The model under review builds one solid part; all positions refer to its coordinate system, in mm. A direction names the side the tool comes from. Coordinates: 2 decimals unless noted, no trailing zeros. Write each loop counter-clockwise with the first axis right and the second up, starting at its lowest first coordinate (ties: lowest second). Pieces come first, ordered by that corner, then holes. Notation, with made-up numbers: (89.5, 57) -> (110.5, 57) arc R24 cw to (110.5, 95) -> close; hole circle Ø7 at (-30, 75). An arc over 180 degrees is marked (long way). Write each question's results on one line, items separated by ' | '.
```python
from build123d import *

# Parameters (mm, degrees)
F1_DEPTH      = 508
F7_DEPTH      = 34.6420161514
F7_DEPTH_BACK = 34.6420161514
F8_DEPTH      = 43.3022701892
F8_DEPTH_BACK = 43.3022701892
F9_DEPTH      = 43.3022701892
F9_DEPTH_BACK = 43.3022701892
F10_R         = 15


with BuildPart() as f1:
    # F0 (on Top) → F1 (new body)
    with BuildSketch(Plane.XY):
        Polygon((17.3205080757, 30), (-17.3205080757, 30), (-34.6410161514, 0), (-17.3205080757, -30), (17.3205080757, -30), (34.6410161514, 0), align=None)
    extrude(amount=F1_DEPTH)

    # F4 (on Right) → F7 (cut, two sides)
    with BuildSketch(Plane.YZ) as f7_sk:
        Polygon((12.4264068712, 60), (30, 42.4264068712), (30, 77.5735931288), align=None)
        Polygon((-30, 77.5735931288), (-30, 42.4264068712), (-12.4264068712, 60), align=None)
        Polygon((12.4264068712, 0), (-12.4264068712, 0), (-30, 17.5735931288), (-30, -5), (30, -5), (30, 17.5735931288), align=None)
    extrude(amount=F7_DEPTH, mode=Mode.SUBTRACT)
    extrude(f7_sk.sketch, amount=-F7_DEPTH_BACK, mode=Mode.SUBTRACT)

    # F5 (on mid) → F8 (cut, two sides)
    with BuildSketch(Plane(origin=(0, 0, 0), x_dir=(-0.8660254038, -0.5, 0), z_dir=(-0.5, 0.8660254038, 0))) as f8_sk:
        Polygon((12.4264068712, 60), (30, 42.4264068712), (30, 77.5735931288), align=None)
        Polygon((-30, 77.5735931288), (-30, 42.4264068712), (-12.4264068712, 60), align=None)
        Polygon((12.4264068712, 0), (-12.4264068712, 0), (-30, 17.5735931288), (-30, -5), (30, -5), (30, 17.5735931288), align=None)
    extrude(amount=F8_DEPTH, mode=Mode.SUBTRACT)
    extrude(f8_sk.sketch, amount=-F8_DEPTH_BACK, mode=Mode.SUBTRACT)

    # F6 (on mid) → F9 (cut, two sides)
    with BuildSketch(Plane(origin=(0, 0, 0), x_dir=(-0.8660254038, 0.5, 0), z_dir=(0.5, 0.8660254038, 0))) as f9_sk:
        Polygon((12.4264068712, 60), (30, 42.4264068712), (30, 77.5735931288), align=None)
        Polygon((-30, 77.5735931288), (-30, 42.4264068712), (-12.4264068712, 60), align=None)
        Polygon((12.4264068712, 0), (-12.4264068712, 0), (-30, 17.5735931288), (-30, -5), (30, -5), (30, 17.5735931288), align=None)
    extrude(amount=F9_DEPTH, mode=Mode.SUBTRACT)
    extrude(f9_sk.sketch, amount=-F9_DEPTH_BACK, mode=Mode.SUBTRACT)

    # F10
    f10_edges = [f1.edges().sort_by_distance(p)[0] for p in [
        (-25.980762, -15, 17.573593),
        (0, -30, 17.573593),
        (25.980762, -15, 17.573593),
        (25.980762, 15, 17.573593),
        (0, 30, 17.573593),
        (-25.980762, 15, 17.573593),
        (25.980762, 15, 42.426407),
        (25.980762, -15, 42.426407),
        (0, 30, 42.426407),
        (-25.980762, 15, 42.426407),
        (0, -30, 42.426407),
        (-25.980762, -15, 42.426407),
        (0, -12.426407, 0),
        (10.761584, -6.213203, 0),
        (10.761584, 6.213203, 0),
        (0, 12.426407, 0),
        (-10.761584, 6.213203, 0),
        (-10.761584, -6.213203, 0),
    ]]
    fillet(f10_edges, radius=F10_R)


solid = f1.part
```
Q1. Draft analysis for pull direction Z (two halves, no side actions). For faces 5 (the flat face through (25.86, -15.21, 289.77)), 6 (the cylindrical face through (-25.14, -14.23, 41.88)), 7 (the cylindrical face through (-0.14, 13.07, 1.66)), state which applies: pulls with the +Z half, pulls with the -Z half, needs draft (parallel to the pull), parting line crosses it, or undercut.
Solution:
face 5: needs draft | face 6: undercut | face 7: pulls with the -Z half
Q2. For line 1 (Z direction, x = -10, y = -21.5); line 2 (Z direction, x = 19.5, y = -13.5); line 3 (Y direction, x = -30.5, z = 334), list the stretches that pass through material, from the lowest coordinate up. Write a range as from..to.
Solution:
line 1: 9.07..50.93, 69.07..508 | line 2: 11.21..48.79, 71.21..508 | line 3: -7.17..7.17
Q3. Clearance check with flat-ended pins moving along their axes: P1, Ø10, axis at y = -13.5, z = 133.5, coming from the -X side; P2, Ø3, axis at y = -7, z = 260, coming from the +X side; P3, Ø1.5, axis at x = -23.5, y = -3, coming from the -Z side. State where each tip first meets the part, or that it passes through.
Solution:
P1: x = -29.73 | P2: x = 31.47 | P3: z = 8.68
Q4. Machinability: for faces 1 (the cylindrical face through (-24.843, 14.623, 42.03)), 2 (the cylindrical face through (24.9, -14.65, 41.88)), 3 (the flat face through (-20.05, -11.85, 70.86)), 4 (the flat face through (20.08, 11.31, 70.62)), which of the approach directions +Z, -Z, +X, -X, +Y, -Y give a long, thin tool a straight path to every point of the face, cutting with its end or side? Answer none if there is none.
Solution:
face 1: -X, +Y | face 2: +X, -Y | face 3: -X, -Y | face 4: +X, +Y
Q5. Add section A-A (z = 84). Write out the cut boundary in (x, y), plus the area to 3 significant figures.
Solution:
outline: (-34.64, 0) -> (-17.32, -30) -> (17.32, -30) -> (34.64, 0) -> (17.32, 30) -> (-17.32, 30) -> close | area: 3,120 mm²
